```python
from build123d import *

# Parameters (mm, degrees)
SKETCH1_W                  = 282
SKETCH1_H                  = 480
BOSS_EXTRUDE1_DEPTH        = 3
CUT_EXTRUDE1_REACH         = 558.716
SKETCH2_R                  = 70
SKETCH2_R_2                = 28.5
SKETCH2_R_3                = 25
SKETCH2_R_4                = 26
SKETCH2_R_5                = 11.5
SKETCH2_R_6                = 11.25
F_4_5_4_5_DIAMETER_HOLE1_D = 4.5
F_4_0_4_DIAMETER_HOLE1_D   = 4


with BuildPart() as part:
    # Sketch1 → Boss-Extrude1 (new body)
    with BuildSketch(Plane(origin=(0, 0, 0), x_dir=(1, 0, 0), z_dir=(0, 1, 0))):
        with Locations((141, 240)):
            Rectangle(SKETCH1_W, SKETCH1_H)
    extrude(amount=BOSS_EXTRUDE1_DEPTH)

    # Sketch2 → Cut-Extrude1 (cut, up to next)
    with BuildSketch(Plane(origin=(0, 3, 0), x_dir=(1, 0, 0), z_dir=(0, 1, 0)), mode=Mode.PRIVATE) as cut_extrude1_sk1:
        with Locations(Location((171, 371.5, 0), (0, 0, 270))):
            Circle(SKETCH2_R)
    cut_extrude1_tool1 = extrude(cut_extrude1_sk1.sketch, amount=-CUT_EXTRUDE1_REACH, mode=Mode.PRIVATE) & part.part
    # Sketch2 → Cut-Extrude1 (cut, up to next)
    with BuildSketch(Plane(origin=(0, 3, 0), x_dir=(1, 0, 0), z_dir=(0, 1, 0)), mode=Mode.PRIVATE) as cut_extrude1_sk2:
        with Locations(Location((61, 330, 0), (0, 0, 270))):
            Circle(SKETCH2_R_2)
    cut_extrude1_tool2 = extrude(cut_extrude1_sk2.sketch, amount=-CUT_EXTRUDE1_REACH, mode=Mode.PRIVATE) & part.part
    # Sketch2 → Cut-Extrude1 (cut, up to next)
    with BuildSketch(Plane(origin=(0, 3, 0), x_dir=(1, 0, 0), z_dir=(0, 1, 0)), mode=Mode.PRIVATE) as cut_extrude1_sk3:
        with Locations(Location((231, 165, 0), (0, 0, 270))):
            Circle(SKETCH2_R_3)
    cut_extrude1_tool3 = extrude(cut_extrude1_sk3.sketch, amount=-CUT_EXTRUDE1_REACH, mode=Mode.PRIVATE) & part.part
    # Sketch2 → Cut-Extrude1 (cut, up to next)
    with BuildSketch(Plane(origin=(0, 3, 0), x_dir=(1, 0, 0), z_dir=(0, 1, 0)), mode=Mode.PRIVATE) as cut_extrude1_sk4:
        with Locations(Location((171, 165, 0), (0, 0, 270))):
            Circle(SKETCH2_R_4)
    cut_extrude1_tool4 = extrude(cut_extrude1_sk4.sketch, amount=-CUT_EXTRUDE1_REACH, mode=Mode.PRIVATE) & part.part
    # Sketch2 → Cut-Extrude1 (cut, up to next)
    with BuildSketch(Plane(origin=(0, 3, 0), x_dir=(1, 0, 0), z_dir=(0, 1, 0)), mode=Mode.PRIVATE) as cut_extrude1_sk5:
        with Locations(Location((111, 165, 0), (0, 0, 270))):
            Circle(SKETCH2_R_4)
    cut_extrude1_tool5 = extrude(cut_extrude1_sk5.sketch, amount=-CUT_EXTRUDE1_REACH, mode=Mode.PRIVATE) & part.part
    # Sketch2 → Cut-Extrude1 (cut, up to next)
    with BuildSketch(Plane(origin=(0, 3, 0), x_dir=(1, 0, 0), z_dir=(0, 1, 0)), mode=Mode.PRIVATE) as cut_extrude1_sk6:
        with Locations(Location((51, 165, 0), (0, 0, 270))):
            Circle(SKETCH2_R_4)
    cut_extrude1_tool6 = extrude(cut_extrude1_sk6.sketch, amount=-CUT_EXTRUDE1_REACH, mode=Mode.PRIVATE) & part.part
    # Sketch2 → Cut-Extrude1 (cut, up to next)
    with BuildSketch(Plane(origin=(0, 3, 0), x_dir=(1, 0, 0), z_dir=(0, 1, 0)), mode=Mode.PRIVATE) as cut_extrude1_sk7:
        with Locations(Location((41, 225, 0), (0, 0, 270))):
            Circle(SKETCH2_R_5)
    cut_extrude1_tool7 = extrude(cut_extrude1_sk7.sketch, amount=-CUT_EXTRUDE1_REACH, mode=Mode.PRIVATE) & part.part
    # Sketch2 → Cut-Extrude1 (cut, up to next)
    with BuildSketch(Plane(origin=(0, 3, 0), x_dir=(1, 0, 0), z_dir=(0, 1, 0)), mode=Mode.PRIVATE) as cut_extrude1_sk8:
        with Locations(Location((76, 225, 0), (0, 0, 270))):
            Circle(SKETCH2_R_5)
    cut_extrude1_tool8 = extrude(cut_extrude1_sk8.sketch, amount=-CUT_EXTRUDE1_REACH, mode=Mode.PRIVATE) & part.part
    # Sketch2 → Cut-Extrude1 (cut, up to next)
    with BuildSketch(Plane(origin=(0, 3, 0), x_dir=(1, 0, 0), z_dir=(0, 1, 0)), mode=Mode.PRIVATE) as cut_extrude1_sk9:
        with Locations(Location((111, 225, 0), (0, 0, 270))):
            Circle(SKETCH2_R_5)
    cut_extrude1_tool9 = extrude(cut_extrude1_sk9.sketch, amount=-CUT_EXTRUDE1_REACH, mode=Mode.PRIVATE) & part.part
    # Sketch2 → Cut-Extrude1 (cut, up to next)
    with BuildSketch(Plane(origin=(0, 3, 0), x_dir=(1, 0, 0), z_dir=(0, 1, 0)), mode=Mode.PRIVATE) as cut_extrude1_sk10:
        with Locations(Location((76, 270, 0), (0, 0, 270))):
            Circle(SKETCH2_R_5)
    cut_extrude1_tool10 = extrude(cut_extrude1_sk10.sketch, amount=-CUT_EXTRUDE1_REACH, mode=Mode.PRIVATE) & part.part
    # Sketch2 → Cut-Extrude1 (cut, up to next)
    with BuildSketch(Plane(origin=(0, 3, 0), x_dir=(1, 0, 0), z_dir=(0, 1, 0)), mode=Mode.PRIVATE) as cut_extrude1_sk11:
        with Locations(Location((151, 270, 0), (0, 0, 270))):
            Circle(SKETCH2_R_5)
    cut_extrude1_tool11 = extrude(cut_extrude1_sk11.sketch, amount=-CUT_EXTRUDE1_REACH, mode=Mode.PRIVATE) & part.part
    # Sketch2 → Cut-Extrude1 (cut, up to next)
    with BuildSketch(Plane(origin=(0, 3, 0), x_dir=(1, 0, 0), z_dir=(0, 1, 0)), mode=Mode.PRIVATE) as cut_extrude1_sk12:
        with Locations(Location((191, 225, 0), (0, 0, 270))):
            Circle(SKETCH2_R_5)
    cut_extrude1_tool12 = extrude(cut_extrude1_sk12.sketch, amount=-CUT_EXTRUDE1_REACH, mode=Mode.PRIVATE) & part.part
    # Sketch2 → Cut-Extrude1 (cut, up to next)
    with BuildSketch(Plane(origin=(0, 3, 0), x_dir=(1, 0, 0), z_dir=(0, 1, 0)), mode=Mode.PRIVATE) as cut_extrude1_sk13:
        with Locations(Location((226, 270, 0), (0, 0, 270))):
            Circle(SKETCH2_R_5)
    cut_extrude1_tool13 = extrude(cut_extrude1_sk13.sketch, amount=-CUT_EXTRUDE1_REACH, mode=Mode.PRIVATE) & part.part
    # Sketch2 → Cut-Extrude1 (cut, up to next)
    with BuildSketch(Plane(origin=(0, 3, 0), x_dir=(1, 0, 0), z_dir=(0, 1, 0)), mode=Mode.PRIVATE) as cut_extrude1_sk14:
        with Locations(Location((226, 225, 0), (0, 0, 270))):
            Circle(SKETCH2_R_5)
    cut_extrude1_tool14 = extrude(cut_extrude1_sk14.sketch, amount=-CUT_EXTRUDE1_REACH, mode=Mode.PRIVATE) & part.part
    # Sketch2 → Cut-Extrude1 (cut, up to next)
    with BuildSketch(Plane(origin=(0, 3, 0), x_dir=(1, 0, 0), z_dir=(0, 1, 0)), mode=Mode.PRIVATE) as cut_extrude1_sk15:
        with Locations(Location((151, 225, 0), (0, 0, 270))):
            Circle(SKETCH2_R_6)
    cut_extrude1_tool15 = extrude(cut_extrude1_sk15.sketch, amount=-CUT_EXTRUDE1_REACH, mode=Mode.PRIVATE) & part.part
    add(cut_extrude1_tool1.solids().sort_by_distance((171, 3, -371.5))[0], mode=Mode.SUBTRACT)
    add(cut_extrude1_tool2.solids().sort_by_distance((61, 3, -330))[0], mode=Mode.SUBTRACT)
    add(cut_extrude1_tool3.solids().sort_by_distance((231, 3, -165))[0], mode=Mode.SUBTRACT)
    add(cut_extrude1_tool4.solids().sort_by_distance((171, 3, -165))[0], mode=Mode.SUBTRACT)
    add(cut_extrude1_tool5.solids().sort_by_distance((111, 3, -165))[0], mode=Mode.SUBTRACT)
    add(cut_extrude1_tool6.solids().sort_by_distance((51, 3, -165))[0], mode=Mode.SUBTRACT)
    add(cut_extrude1_tool7.solids().sort_by_distance((41, 3, -225))[0], mode=Mode.SUBTRACT)
    add(cut_extrude1_tool8.solids().sort_by_distance((76, 3, -225))[0], mode=Mode.SUBTRACT)
    add(cut_extrude1_tool9.solids().sort_by_distance((111, 3, -225))[0], mode=Mode.SUBTRACT)
    add(cut_extrude1_tool10.solids().sort_by_distance((76, 3, -270))[0], mode=Mode.SUBTRACT)
    add(cut_extrude1_tool11.solids().sort_by_distance((151, 3, -270))[0], mode=Mode.SUBTRACT)
    add(cut_extrude1_tool12.solids().sort_by_distance((191, 3, -225))[0], mode=Mode.SUBTRACT)
    add(cut_extrude1_tool13.solids().sort_by_distance((226, 3, -270))[0], mode=Mode.SUBTRACT)
    add(cut_extrude1_tool14.solids().sort_by_distance((226, 3, -225))[0], mode=Mode.SUBTRACT)
    add(cut_extrude1_tool15.solids().sort_by_distance((151, 3, -225))[0], mode=Mode.SUBTRACT)

    # Ø4.5 (4.5) Diameter Hole1 (through all)
    with Locations(Plane(origin=(0, 0, 0), x_dir=(-1, 0, 0), z_dir=(0, -1, 0))):
        with Locations((-272, 450), (-272, 345), (-272, 240), (-272, 135), (-272, 30), (-10, 345), (-10, 240), (-10, 135), (-10, 30), (-10, 450)):
            Hole(F_4_5_4_5_DIAMETER_HOLE1_D / 2)

    # Ø4.0 (4) Diameter Hole1 (through all)
    with Locations(Plane(origin=(0, 0, 0), x_dir=(-1, 0, 0), z_dir=(0, -1, 0))):
        with Locations((-84.68807717, 353.68807717), (-37.31192283, 353.68807717), (-37.31192283, 306.31192283), (-84.68807717, 306.31192283)):
            Hole(F_4_0_4_DIAMETER_HOLE1_D / 2)


solid = part.part
```
CAD build for the part. Positions are in the model's coordinates, mm. Coordinates: 2 decimals unless noted, no trailing zeros. Order: outer loops, then holes, each group sorted by start corner. A loop starts at its lowest first (then second) coordinate and runs counter-clockwise, first axis right, second up. Notation, with made-up numbers: (60, 72.5) - (111, 72.5) arc R24 cw to (111, 109.5) - close; hole circle Ø2 at (89, 6). An arc over 180 degrees is marked (long way). Answer in a Markdown table with one row per item.
1. Slice it at A-A, the plane z = -225. List the corners of the cut face in (x, y), then the cut area to 4 significant figures.
Answer:
| item | result |
|---|---|
| outline | (0, 0) - (29.5, 0) - (29.5, 3) - (0, 3) - close; (52.5, 0) - (64.5, 0) - (64.5, 3) - (52.5, 3) - close; (87.5, 0) - (99.5, 0) - (99.5, 3) - (87.5, 3) - close; (122.5, 0) - (139.75, 0) - (139.75, 3) - (122.5, 3) - close; (162.25, 0) - (179.5, 0) - (179.5, 3) - (162.25, 3) - close; (202.5, 0) - (214.5, 0) - (214.5, 3) - (202.5, 3) - close; (237.5, 0) - (282, 0) - (282, 3) - (237.5, 3) - close |
| area | 433.5 mm² |
2. Slice it at B-B, the plane x = 191. List the corners of the cut face in (y, z).
Answer:
| item | result |
|---|---|
| outline | (0, -480) - (3, -480) - (3, -438.58) - (0, -438.58) - close; (0, -304.42) - (3, -304.42) - (3, -236.5) - (0, -236.5) - close; (0, -213.5) - (3, -213.5) - (3, -181.61) - (0, -181.61) - close; (0, -148.39) - (3, -148.39) - (3, 0) - (0, 0) - close |
3. Slice it at D-D, the plane y = 0.6. Give the number of separate pieces and of enclosed holes in the cut face, then the cut area to 3 significant figures.
Answer:
| item | result |
|---|---|
| separate pieces | 1 |
| enclosed holes | 29 |
| area | 105,000 mm² |
4. Drill centre lines: L1, parallel to X at y = 1, z = -165; L2, parallel to X at y = 2, z = -330; L3, parallel to Z at x = 249.5, y = 1.15. Where is each one in solid material? Low to high. Write a range as from..to.
Answer:
| item | result |
|---|---|
| L1 | 0..25, 77..85, 137..145, 197..206, 256..282 |
| L2 | 0..32.5, 89.5..114.63, 227.37..282 |
| L3 | -480..-181.82, -148.18..0 |
5. Pull direction X, two halves, no side cores. Call faces 1 (the face through (139, 0, -243)), 2 (the face through (71.595, 1.521, -259.377)): +X half, -X half, draft (parallel to the pull), parting line (faces both ways), or undercut.
Answer:
| item | result |
|---|---|
| face 1 | draft |
| face 2 | undercut |
6. Slice it at C-C, the plane z = -320. List the corners of the cut face in (x, y).
Answer:
| item | result |
|---|---|
| outline | (0, 0) - (34.31, 0) - (34.31, 3) - (0, 3) - close; (87.69, 0) - (123.59, 0) - (123.59, 3) - (87.69, 3) - close; (218.41, 0) - (282, 0) - (282, 3) - (218.41, 3) - close |
7. Flat gauge pin, fed straight in: P1, Ø2.5, axis at x = 84.69, z = -353.69, coming from the -Y side. Where does the tip first touch, or does it go through?
Answer:
| item | result |
|---|---|
| P1 | through |
